```python
from build123d import *

# Parameters (mm, degrees)
F0_W             = 80
F0_H             = 187
F1_DEPTH         = 3
F2_W             = 80
F2_H             = 3
F3_DEPTH         = 100
F5_DEPTH         = 3
F7_DEPTH         = 10
F8_W             = 13
F8_H             = 2.5
F9_DEPTH         = 3
F10_R            = 10
F11_R            = 5
F13_DEPTH        = 10
F16_D            = 3.75
F16_DEPTH        = 4.5
F16_TIP          = 1.1266136607
F16_ON_F15_D     = 3.75
F16_ON_F15_DEPTH = 4.5
F16_ON_F15_TIP   = 1.1266136607


with BuildPart() as f1:
    # F0 (on Top) → F1 (new body)
    with BuildSketch(Plane.XY):
        with Locations((-40, 0)):
            Rectangle(F0_W, F0_H)
    extrude(amount=F1_DEPTH)

    # F2 (on face) → F3 (join)
    with BuildSketch(Plane.XY.offset(3)):
        with Locations((-40, 92)):
            Rectangle(F2_W, F2_H)
    extrude(amount=F3_DEPTH)

    # F4 (on face) → F5 (join)
    with BuildSketch(Plane(origin=(-80, 0, 0), x_dir=(0, -1, 0), z_dir=(-1, 0, 0))):
        Polygon((-90.5, 90), (-90.5, 3), (93.5, 3), (93.5, 23), (73.5, 23), (73.5, 87), align=None)
    extrude(amount=-F5_DEPTH)

    # F6 (on face) → F7 (join)
    with BuildSketch(Plane.YZ.offset(-77)):
        Polygon((-71, 86.5415299445), (-73.5, 87), (-73.5, 23), (-71, 23), align=None)
    extrude(amount=F7_DEPTH)

    # F8 (on face) → F9 (join)
    with BuildSketch(Plane.XZ.offset(73.5)):
        with Locations((-73.5, 85.75)):
            Rectangle(F8_W, F8_H)
    extrude(amount=F9_DEPTH)

    # F10
    f10_edges = [f1.edges().sort_by_distance(p)[0] for p in [
        (-80, 92, 103),
    ]]
    fillet(f10_edges, radius=F10_R)

    # F11
    f11_edges = [f1.edges().sort_by_distance(p)[0] for p in [
        (-67, -72.25, 23),
    ]]
    fillet(f11_edges, radius=F11_R)

    # F12 (on face) → F13 (join)
    with BuildSketch(Plane.YZ):
        Polygon((93.5, 0), (93.5, 103), (92, 103), (92, 1.5), (-93.5, 1.5), (-93.5, 0), align=None)
    extrude(amount=F13_DEPTH)

    # F16
    with Locations(Plane.XY.offset(1.5)):
        with Locations((5, -60), (5, 0), (5, 60)):
            Hole(F16_D / 2, depth=F16_DEPTH)
            with Locations((0, 0, -(F16_DEPTH + F16_TIP / 2))):  # 118° drill point
                Cone(0, F16_D / 2, F16_TIP, mode=Mode.SUBTRACT)

    # F16 on F15
    with Locations(Plane.XZ.offset(-92)):
        with Locations((5, 25), (5, 91)):
            Hole(F16_ON_F15_D / 2, depth=F16_ON_F15_DEPTH)
            with Locations((0, 0, -(F16_ON_F15_DEPTH + F16_ON_F15_TIP / 2))):  # 118° drill point
                Cone(0, F16_ON_F15_D / 2, F16_ON_F15_TIP, mode=Mode.SUBTRACT)


solid = f1.part
```
CAD build for the part. Positions are in the model's coordinates, mm. A direction names the side the tool comes from. Round coordinates to 2 decimals unless told otherwise and drop trailing zeros. Order: outer loops, then holes, each group sorted by start corner. A loop starts at its lowest first (then second) coordinate and runs counter-clockwise, first axis right, second up.
Item 1: Saw through at B-B on x = 5. Write the cut outline in (y, z) (3 decimals).
Item 2: Mould opens along Z. For faces 1 (the face through (-68, -72, 25)), 2 (the face through (-77.15, 92.02, 99.99)), 3 (the face through (-36, 93.5, 51)) say: pulls with the +Z half, pulls with the -Z half, needs draft (parallel to the pull), parting line crosses it, or undercut.
Item 3: Probe line 1 along Z through (x, y) = (5, 93) (3 decimals); line 2 along Y through (x, z) = (5, 0.6) (3 decimals); line 3 along Y through (x, z) = (-72.5, 32). List the from-to ranges inside material, lowest first.
Item 4: Tool access for faces 4 (the face through (5, 92, 53)), 5 (the face through (-41, 90.5, 52)), 6 (the face through (-74, -73.5, 54)), 7 (the face through (-80, 1, 46)): list every direction of +Z, -Z, +X, -X, +Y, -Y with a clear straight run to the whole face (end or side of a thin tool).
Item 5: Saw through at A-A on z = 25. Write the cut outline in (x, y) (3 decimals), then the cut area to 3 significant figures.
Item 6: Saw through at D-D on z = 49.5. Write the cut outline in (x, y), then the cut area to 3 significant figures.
Item 7: Pin check, flat tips, straight feed: pin 1 (6 mm diameter, centred on y = -72.5, z = 54, fed in from +X); pin 2 (1 mm diameter, centred on x = -16, y = -49, fed in from +Z); pin 3 (3 mm diameter, centred on x = -72.5, z = 86, fed in from -Y). Stop position of each tip, or through.
Item 8: Saw through at C-C on y = -60. Write the cut outline in (x, z) (3 decimals).
Reported:
1. outline: (-93.5, 0) - (-61.875, 0) - (-61.875, 1.5) - (-93.5, 1.5) - close; (-58.125, 0) - (-1.875, 0) - (-1.875, 1.5) - (-58.125, 1.5) - close; (1.875, 0) - (58.125, 0) - (58.125, 1.5) - (1.875, 1.5) - close; (61.875, 0) - (93.5, 0) - (93.5, 23.125) - (92, 23.125) - (92, 1.5) - (61.875, 1.5) - close; (92, 26.875) - (93.5, 26.875) - (93.5, 89.125) - (92, 89.125) - close; (92, 92.875) - (93.5, 92.875) - (93.5, 103) - (92, 103) - close
2. face 1: undercut
2. face 2: pulls with the +Z half
2. face 3: needs draft
3. line 1: z = 0 to 23.125, 26.875 to 89.125, 92.875 to 103
3. line 2: y = -93.5 to -61.875, -58.125 to -1.875, 1.875 to 58.125, 61.875 to 93.5
3. line 3: y = -73.5 to -71, 90.5 to 93.5
4. face 4: +Z, +X, -Y
4. face 5: +Z, +X
4. face 6: +X, -X, -Y
4. face 7: +Z, -Z, -X, +Y, -Y
5. outline: (-80, -73.5) - (-68, -73.5) - (-68, -71) - (-77, -71) - (-77, 90.5) - (0, 90.5) - (0, 92) - (3.125, 92) - (3.125, 93.5) - (-80, 93.5) - close; (6.875, 92) - (10, 92) - (10, 93.5) - (6.875, 93.5) - close
5. area: 764 mm2
6. outline: (-80, -73.5) - (-67, -73.5) - (-67, -71) - (-77, -71) - (-77, 90.5) - (0, 90.5) - (0, 92) - (10, 92) - (10, 93.5) - (-80, 93.5) - close
6. area: 772 mm2
7. pin 1: stops at x = -67
7. pin 2: stops at z = 3
7. pin 3: stops at y = -76.5
8. outline: (-80, 0) - (3.125, 0) - (3.125, 1.5) - (0, 1.5) - (0, 3) - (-77, 3) - (-77, 87.247) - (-80, 87.247) - close; (6.875, 0) - (10, 0) - (10, 1.5) - (6.875, 1.5) - close
